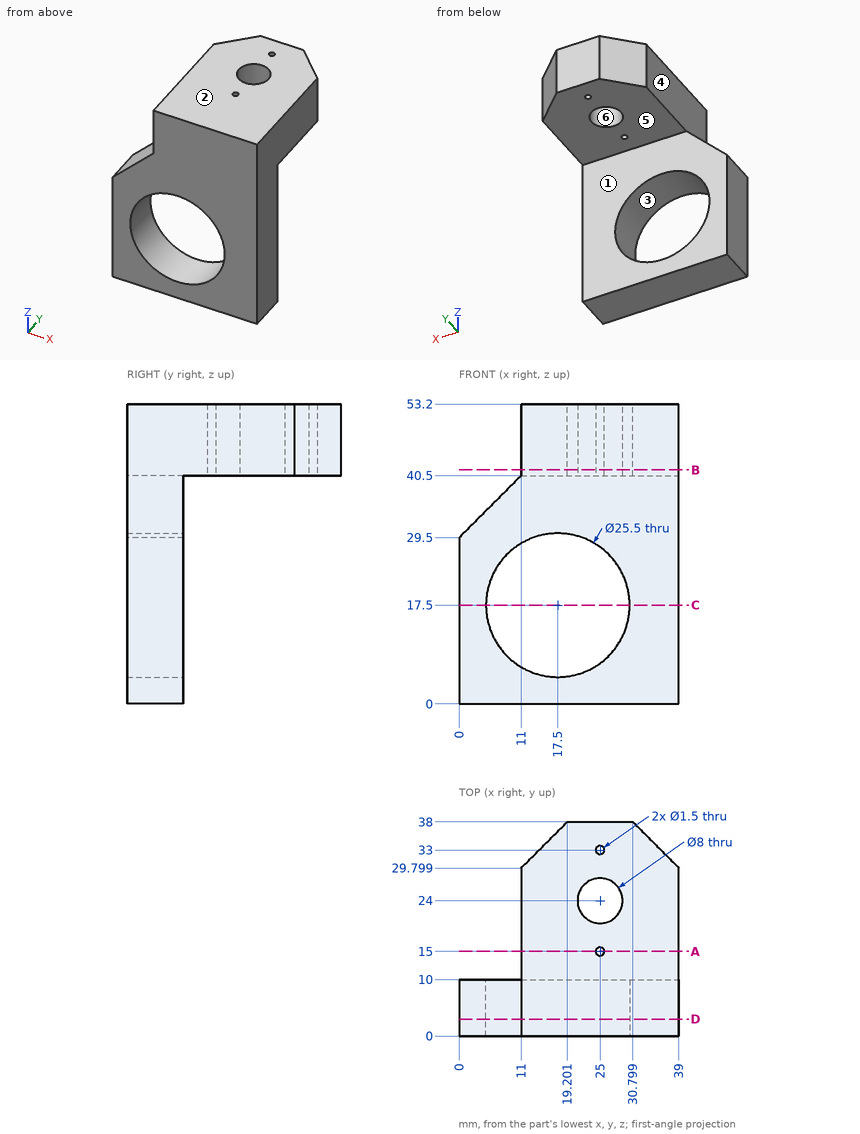
The drawing under review shows one solid part. Ordinate dimensions are in mm from its lowest x, y, z. A direction names the side the tool comes from. Round coordinates to 2 decimals unless told otherwise and drop trailing zeros. Write each loop counter-clockwise with the first axis right and the second up, starting at its lowest first coordinate (ties: lowest second). Pieces come first, ordered by that corner, then holes. Notation, with made-up numbers: (17.5, 14.25) -> (51.5, 14.25) arc R8 cw to (51.5, 28.25) -> close; hole circle Ø8 at (53, -36.5). An arc over 180 degrees is marked (long way). Put each result on its own line as item: value.
Q1. To check wall thickness, follow L1, parallel to Z at x = 17.5, y = 2.25; L2, parallel to Y at x = 25, z = 48; L3, parallel to X at y = 9, z = 17. State the ranges of each line that lie inside material, in increasing order. Write a range as [from, to].
Determined:
L1: z = [0, 4.75], [30.25, 53.2]
L2: y = [0, 14.25], [15.75, 20], [28, 32.25], [33.75, 38]
L3: x = [0, 4.76], [30.24, 39]
Q2. Consider section B-B on z = 41.5. State the section outline as (x, y) points, and give its area (3 significant figures).
Determined:
outline: (11, 0) -> (39, 0) -> (39, 29.8) -> (30.8, 38) -> (19.2, 38) -> (11, 29.8) -> close; hole circle Ø8 at (25, 24); hole circle Ø1.5 at (25, 15); hole circle Ø1.5 at (25, 33)
area: 943 mm^2
Q3. Consider section A-A on y = 15. State the section outline as (x, z) points.
Determined:
outline: (11, 40.5) -> (24.25, 40.5) -> (24.25, 53.2) -> (11, 53.2) -> close; (25.75, 40.5) -> (39, 40.5) -> (39, 53.2) -> (25.75, 53.2) -> close
Q4. The part is to be moulded in two halves that separate along Z. For the marked faces 1, 2 and 3, say which applies: released by +Z, released by -Z, zero draft, split by the parting line, or undercut.
Determined:
face 1: zero draft
face 2: released by +Z
face 3: undercut
Q5. Consider section C-C on z = 17.5. State the section outline as (x, y) points.
Determined:
outline: (0, 0) -> (4.75, 0) -> (4.75, 10) -> (0, 10) -> close; (30.25, 0) -> (39, 0) -> (39, 10) -> (30.25, 10) -> close
Q6. Machinability: for the marked faces 4, 5 and 6, which of the approach directions +Z, -Z, +X, -X, +Y, -Y give a long, thin tool a straight path to every point of the face, cutting with its end or side? Answer none if there is none.
Determined:
face 4: +Z, -X, +Y, -Y
face 5: -Z, +X, -X, +Y
face 6: +Z, -Z
Q7. Consider section D-D on y = 3. State the section outline as (x, z) points, and give its area (3 significant figures).
Determined:
outline: (0, 0) -> (39, 0) -> (39, 53.2) -> (11, 53.2) -> (11, 40.5) -> (0, 29.5) -> close; hole circle Ø25.5 at (17.5, 17.5)
area: 1,360 mm^2
Q8. Clearance check with flat-ended pins moving along their axes: pin 1 Ø1.5 at (y, z) = (16.5, 41.5) entering from -X; pin 2 Ø14 at (x, y) = (20.5, 29.5) entering from -Z. State where each tip first meets the part, or that it passes through.
Determined:
pin 1: stops at x = 11
pin 2: stops at z = 40.5
